CAD build for the part. Positions are in the model's coordinates, mm. Face numbers are marked on the shaded views. Give positions to 0.01 mm unless a question says otherwise; leave off trailing zeros. Write each loop counter-clockwise with the first axis right and the second up, starting at its lowest first coordinate (ties: lowest second). Pieces come first, ordered by that corner, then holes. Notation, with made-up numbers: (-40, 36) - (-11, 36) arc R27 cw to (-11, 68) - close; hole circle Ø5 at (51.5, -12.75). An arc over 180 degrees is marked (long way). Answer as a JSON object with one key per item and string values.
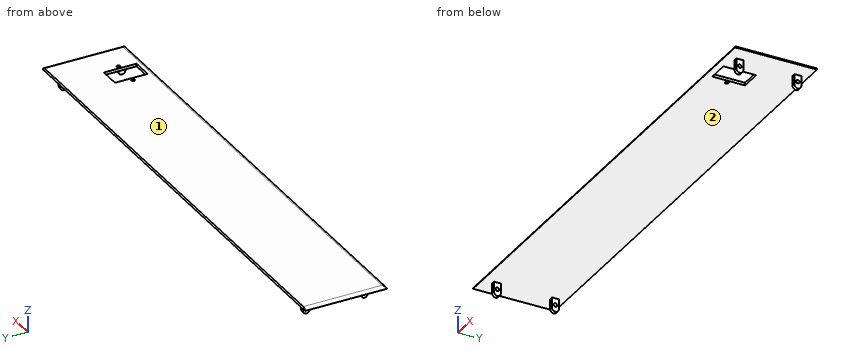
from build123d import *

# Parameters (mm, degrees)
SKETCH1_W              = 708
SKETCH1_H              = 120
BOSS_EXTRUDE1_DEPTH    = 4
CUT_EXTRUDE1_REACH     = 720.109
SKETCH2_R              = 2.55
SKETCH2_W              = 30
SKETCH2_H              = 48
SKETCH3_W              = 5
SKETCH3_H              = 10
BOSS_EXTRUDE2_DEPTH    = 20
SKETCH4_R              = 2.6
CUT_EXTRUDE2_DEPTH     = 20
FILLET1_R              = 5
LPATTERN1_COUNT        = 2
LPATTERN1_PITCH        = 85
FILLET1_OF_LPATTERN1_R = 5
MIRROR5_START          = 24
MIRROR5_OUTLINE_R      = 2.6
MIRROR5_DEPTH          = 5
FILLET2_R              = 5


# Read off the part's stored shape, not the designer's step: Mirror5
# Some blends are built 0.0001 mm under size
with BuildPart() as part:
    # Sketch1 → Boss-Extrude1 (new body)
    with BuildSketch(Plane.XY):
        with Locations((354, 60)):
            Rectangle(SKETCH1_W, SKETCH1_H)
    extrude(amount=BOSS_EXTRUDE1_DEPTH)

    # Sketch2 → Cut-Extrude1 (cut, up to next)
    with BuildSketch(Plane.XY.offset(4), mode=Mode.PRIVATE) as cut_extrude1_sk1:
        with Locations((623, 34)):
            Circle(SKETCH2_R)
    cut_extrude1_tool1 = extrude(cut_extrude1_sk1.sketch, amount=-CUT_EXTRUDE1_REACH, mode=Mode.PRIVATE) & part.part
    # Sketch2 → Cut-Extrude1 (cut, up to next)
    with BuildSketch(Plane.XY.offset(4), mode=Mode.PRIVATE) as cut_extrude1_sk2:
        with Locations((663, 34)):
            Circle(SKETCH2_R)
    cut_extrude1_tool2 = extrude(cut_extrude1_sk2.sketch, amount=-CUT_EXTRUDE1_REACH, mode=Mode.PRIVATE) & part.part
    # Sketch2 → Cut-Extrude1 (cut, up to next)
    with BuildSketch(Plane.XY.offset(4), mode=Mode.PRIVATE) as cut_extrude1_sk3:
        with Locations((643, 34)):
            Rectangle(SKETCH2_W, SKETCH2_H)
    cut_extrude1_tool3 = extrude(cut_extrude1_sk3.sketch, amount=-CUT_EXTRUDE1_REACH, mode=Mode.PRIVATE) & part.part
    add(cut_extrude1_tool1.solids().sort_by_distance((623, 34, 4))[0], mode=Mode.SUBTRACT)
    add(cut_extrude1_tool2.solids().sort_by_distance((663, 34, 4))[0], mode=Mode.SUBTRACT)
    add(cut_extrude1_tool3.solids().sort_by_distance((643, 34, 4))[0], mode=Mode.SUBTRACT)

    # Sketch3 → Boss-Extrude2 (add)
    with BuildSketch(Plane(origin=(0, 0, 0), x_dir=(-1, 0, 0), z_dir=(0, 0, -1))):
        with Locations((-681.5, 20)):
            Rectangle(SKETCH3_W, SKETCH3_H)
    boss_extrude2 = extrude(amount=BOSS_EXTRUDE2_DEPTH)

    # Sketch4 → Cut-Extrude2 (cut)
    with BuildSketch(Plane(origin=(684, 0, 0), x_dir=(0, 0, -1), z_dir=(1, 0, 0))):
        with Locations((10, 20)):
            Circle(SKETCH4_R)
    cut_extrude2 = extrude(amount=-CUT_EXTRUDE2_DEPTH, mode=Mode.SUBTRACT)

    # Fillet1
    fillet1_edges = [part.edges().sort_by_distance(p)[0] for p in [
        (681.5, 15, -20),
        (681.5, 25, -20),
    ]]
    fillet(fillet1_edges, radius=FILLET1_R - 0.0001)  # a hair under: the kernel refuses the full size

    # LPattern1: Boss-Extrude2, Cut-Extrude2 ×2
    with Locations(*[(0, i * LPATTERN1_PITCH, 0) for i in range(1, LPATTERN1_COUNT)]):
        add(boss_extrude2)
        add(cut_extrude2, mode=Mode.SUBTRACT)

    # Fillet1 of LPattern1
    fillet1_of_lpattern1_edges = [part.edges().sort_by_distance(p)[0] for p in [
        (681.5, 100, -20),
        (681.5, 110, -20),
    ]]
    fillet(fillet1_of_lpattern1_edges, radius=FILLET1_OF_LPATTERN1_R - 0.0001)  # a hair under: the kernel refuses the full size

    # Mirror5 outline → Mirror5 (add)
    # profile 1 of 2: a face of its own
    with BuildSketch(Plane.YZ.offset(MIRROR5_START)):
        with BuildLine():
            Line((25, 0), (15, 0))
            Line((15, 0), (15, -15))
            ThreePointArc((15, -15), (16.464466094, -18.535533906), (20, -20))
            ThreePointArc((20, -20), (23.535533906, -18.535533906), (25, -15))
            Line((25, -15), (25, 0))
        make_face()
        with Locations((20, -10)):
            Circle(MIRROR5_OUTLINE_R, mode=Mode.SUBTRACT)
    # profile 2 of 2: a face of its own
    with BuildSketch(Plane.YZ.offset(MIRROR5_START)):
        with BuildLine():
            Line((110, 0), (100, 0))
            Line((100, 0), (100, -15))
            ThreePointArc((100, -15), (101.464466094, -18.535533906), (105, -20))
            ThreePointArc((105, -20), (108.535533906, -18.535533906), (110, -15))
            Line((110, -15), (110, 0))
        make_face()
        with Locations((105, -10)):
            Circle(MIRROR5_OUTLINE_R, mode=Mode.SUBTRACT)
    extrude(amount=MIRROR5_DEPTH)

    # Fillet2
    # the kernel refuses this fillet: 5 mm, written as the material it takes off along each edge
    with BuildSketch(Plane(origin=(0, 132.247448714, 4), x_dir=(1.5589751711781488e-12, 0, -1.0), z_dir=(0, -1, 0)), Plane(origin=(708, -12.247448714, 4), x_dir=(-1.5631940186717186e-12, 0, -1.0), z_dir=(0, 1, 0))) as fillet2_piece_1:
        with BuildLine():
            CenterArc((5, 4.898979486), FILLET2_R, 180, 78.463040967)
            Line((0, 4.898979486), (-0.1, 4.898979486))
            Line((-0.1, 4.898979486), (-0.1, 0))
            Line((-0.1, 0), (0, -0.1))
            ThreePointArc((0, -0.1), (2, -0.1), (3.98, -0.09797959))
            Line((3.98, -0.09797959), (4, 0))
        make_face()
    extrude(amount=144.494897428, mode=Mode.SUBTRACT)
    with BuildSketch(Plane(origin=(-12.247448714, 0, 4), x_dir=(0, 1.5725198920785669e-12, -1.0), z_dir=(1, 0, 0))) as fillet2_piece_2:
        with BuildLine():
            CenterArc((5, 4.898979486), FILLET2_R, 180, 78.463040967)
            Line((0, 4.898979486), (-0.1, 4.898979486))
            Line((-0.1, 4.898979486), (-0.1, 0))
            Line((-0.1, 0), (0, -0.1))
            ThreePointArc((0, -0.1), (2, -0.1), (3.98, -0.09797959))
            Line((3.98, -0.09797959), (4, 0))
        make_face()
    extrude(amount=732.494897428, mode=Mode.SUBTRACT)


solid = part.part
Item 1: Mould opens along X. For the marked faces 1 and 2 say: +X half, -X half, draft (parallel to the pull), parting line (faces both ways), or undercut.
Entries:
{"face 1": "draft", "face 2": "undercut"}
Item 2: Cut at A-A (y = 47). Give the cut face in (x, z).
Entries:
{"outline": "(0, 0) - (628, 0) - (628, 4) - (4.9, 4) arc R5 ccw to start; (658, 0) - (708, 0) arc R5 ccw to (703.1, 4) - (658, 4) - close"}
Item 3: Cut at B-B (x = 115). Give the cut face in (y, z).
Entries:
{"outline": "(0, 0) - (120, 0) - (120, 4) - (4.9, 4) arc R5 ccw to start"}
Item 4: Flat gauge pins, fed straight in: P1, Ø4, axis at x = 623, y = 34, coming from the -Z side; P2, Ø5.5, axis at x = 681, z = -11, coming from the +Y side; P3, Ø1.5, axis at x = 277, y = 37, coming from the -Z side; P4, Ø3, axis at y = 22, z = -13.5, coming from the +X side. Where does each tip first touch, or does it go through?
Entries:
{"P1": "through", "P2": "y = 110", "P3": "z = 0", "P4": "x = 684"}
Item 5: Probe line 1 (Z direction, x = 147, y = 36); line 2 (Z direction, x = 28, y = 105); line 3 (Y direction, x = 623, z = 1.65). List the from-to ranges inside material, lowest first. Write a range as from..to.
Entries:
{"line 1": "0..4", "line 2": "-20..-12.6, -7.4..4", "line 3": "0.66..31.45, 36.55..120"}
